```python
from build123d import *

# Parameters (mm, degrees)
PAD_DEPTH    = 30
SKETCH001_W  = 15
SKETCH001_H  = 6
PAD001_DEPTH = 21
SKETCH002_R  = 4
POCKET_DEPTH = 6
FILLET_R     = 4
FILLET001_R  = 3
FILLET002_R  = 1
FILLET003_R  = 1


with BuildPart() as part:
    # Sketch → Pad (new body)
    with BuildSketch(Plane.XY):
        Polygon((-17.5, 20), (-17.5, 0), (17.5, 0), (17.5, 20), (20.5, 20), (27.5, -5), (-27.5, -5), (-20.5, 20), align=None)
    extrude(amount=PAD_DEPTH)

    # Sketch001 (on Face1 of Pad) → Pad001 (join)
    with BuildSketch(Plane.YZ.offset(-17.5)):
        with Locations((10, 15)):
            Rectangle(SKETCH001_W, SKETCH001_H)
    extrude(amount=-PAD001_DEPTH)

    # Sketch002 (on Face15 of Pad001) → Pocket (cut)
    with BuildSketch(Plane.XY.offset(18)):
        with Locations((-29.8, 10)):
            Circle(SKETCH002_R)
    extrude(amount=-POCKET_DEPTH, mode=Mode.SUBTRACT)

    # Fillet
    fillet_edges = [part.edges().sort_by_distance(p)[0] for p in [
        (-38.5, 17.5, 15),
        (-38.5, 2.5, 15),
    ]]
    fillet(fillet_edges, radius=FILLET_R)

    # Fillet001
    fillet001_edges = [part.edges().sort_by_distance(p)[0] for p in [
        (-27.5, -5, 15),
        (27.5, -5, 15),
    ]]
    fillet(fillet001_edges, radius=FILLET001_R)

    # Fillet002
    fillet002_edges = [part.edges().sort_by_distance(p)[0] for p in [
        (-20.5, 20, 15),
        (20.5, 20, 15),
    ]]
    fillet(fillet002_edges, radius=FILLET002_R)

    # Fillet003
    fillet003_edges = [part.edges().sort_by_distance(p)[0] for p in [
        (-23.3, 10, 18),
        (-23.3, 10, 12),
        (-21.2, 17.5, 15),
        (-25.4, 2.5, 15),
    ]]
    fillet(fillet003_edges, radius=FILLET003_R)


solid = part.part
```
CAD build for the part. Positions are in the model's coordinates, mm. A direction names the side the tool comes from. Give positions to 0.01 mm unless a question says otherwise; leave off trailing zeros. Order: outer loops, then holes, each group sorted by start corner. A loop starts at its lowest first (then second) coordinate and runs counter-clockwise, first axis right, second up.
(1) Saw through at D-D, the plane y = 7.75. State how many separate pieces and enclosed holes the cut face has, then the cut area to 3 significant figures.
(2) Saw through at B-B, the plane z = 20.25. Give the cut face in (x, y).
(3) Drill centre lines: L1, parallel to Y at x = -29.8, z = 16.55; L2, parallel to Z at x = -26, y = 14.75; L3, parallel to Y at x = 3, z = 26.5. Where is each one in solid material? Low to high.
(4) Mould opens along X. For faces 1 (the cylindrical face through (25.911, -3.844, 15.21)), 2 (the cylindrical face through (-37.297, 3.641, 15.042)), 3 (the cylindrical face through (-25.985, 11.201, 15.042)), 4 (the flat face through (6, -1, 30)) say: released by +X, released by -X, zero draft, split by the parting line, or undercut.
(5) Saw through at A-A, the plane x = -29.8. Give the cut face in (y, z).
(6) Saw through at C-C, the plane z = 13.5. Give the cut face in (x, y), then the cut area to 3 significant figures.
(7) Flat gauge pins, fed straight in: pin 1 (12 mm diameter, centred on x = -32.5, y = 7, fed in from +Z); pin 2 (7 mm diameter, centred on x = -29.8, y = 10, fed in from +Z); pin 3 (2 mm diameter, centred on y = 9.5, z = 10.5, fed in from -X); pin 4 (5 mm diameter, centred on x = -3.5, z = 4.5, fed in from +Y). Where does each tip first touch, or does it go through?
(8) Tool access for faces 5 (the flat face through (-34, 10, 12)), 6 (the flat face through (-31, 2.5, 15)), 7 (the flat face through (-28, 17.5, 15)), 8 (the flat face through (0, 0, 15)): list every direction of +Z, -Z, +X, -X, +Y, -Y with a clear straight run to the whole face (end or side of a thin tool).
Results found:
1. separate pieces: 3
1. enclosed holes: 0
1. area: 434 mm2
2. outline: (-26.43, -1.19) arc R3 ccw to (-23.54, -5) - (23.54, -5) arc R3 ccw to (26.43, -1.19) - (20.7, 19.27) arc R1 ccw to (19.74, 20) - (17.5, 20) - (17.5, 0) - (-17.5, 0) - (-17.5, 20) - (-19.74, 20) arc R1 ccw to (-20.7, 19.27) - close
3. L1: y = 2.5 to 6, 14 to 17.5
3. L2: z = 12 to 18
3. L3: y = -5 to 0
4. face 1: released by +X
4. face 2: released by -X
4. face 3: undercut
4. face 4: zero draft
5. outline: (2.5, 12) - (6, 12) - (6, 18) - (2.5, 18) - close; (14, 12) - (17.5, 12) - (17.5, 18) - (14, 18) - close
6. outline: (-38.5, 6.5) arc R4 ccw to (-34.5, 2.5) - (-26.72, 2.5) arc R1 cw to (-25.76, 1.23) - (-26.43, -1.19) arc R3 ccw to (-23.54, -5) - (23.54, -5) arc R3 ccw to (26.43, -1.19) - (20.7, 19.27) arc R1 ccw to (19.74, 20) - (17.5, 20) - (17.5, 0) - (-17.5, 0) - (-17.5, 20) - (-19.74, 20) arc R1 ccw to (-20.7, 19.27) - (-21, 18.23) arc R1 cw to (-21.96, 17.5) - (-34.5, 17.5) arc R4 ccw to (-38.5, 13.5) - close; hole circle Ø8 at (-29.8, 10)
6. area: 664 mm2
7. pin 1: stops at z = 18
7. pin 2: passes through
7. pin 3: stops at x = -23.72
7. pin 4: stops at y = 0
8. face 5: -Z, -X, +Y
8. face 6: +Z, -Z, -X, -Y
8. face 7: +Z, -Z, -X, +Y
8. face 8: +Z, -Z, +Y
